```python
from build123d import *

# Parameters (mm, degrees)
SKETCH_1_W          = 84
SKETCH_1_H          = 55
EXTRUDE_2_DEPTH     = 8.5
EXTRUDE_3_DEPTH     = 5
SKETCH_2_W          = 84
SKETCH_2_H          = 3
CUT_EXTRUDE_1_DEPTH = 2


with BuildPart() as part:
    # Sketch 1 → Extrude 2 (new body)
    with BuildSketch(Plane.XY):
        Rectangle(SKETCH_1_W, SKETCH_1_H)
    extrude(amount=EXTRUDE_2_DEPTH)

    # Sketch 1_3 → Extrude 3 (add)
    with BuildSketch(Plane.XY):
        with BuildLine():
            Line((-29, 27.5), (-25, 27.5))
            ThreePointArc((-25, 27.5), (-27, 29.5), (-29, 27.5))
        make_face()
        with BuildLine():
            ThreePointArc((-42, 24.5), (-44, 22.5), (-42, 20.5))
            Line((-42, 20.5), (-42, 24.5))
        make_face()
        with BuildLine():
            ThreePointArc((-42, 2), (-44, 0), (-42, -2))
            Line((-42, -2), (-42, 2))
        make_face()
        with BuildLine():
            ThreePointArc((-42, -20.5), (-44, -22.5), (-42, -24.5))
            Line((-42, -24.5), (-42, -20.5))
        make_face()
        with BuildLine():
            Line((25, 27.5), (29, 27.5))
            ThreePointArc((29, 27.5), (27, 29.5), (25, 27.5))
        make_face()
    extrude(amount=EXTRUDE_3_DEPTH)

    # Sketch 2 → Cut-Extrude 1 (cut)
    with BuildSketch(Plane.XY.offset(8.5)):
        Rectangle(SKETCH_2_W, SKETCH_2_H)
    extrude(amount=-CUT_EXTRUDE_1_DEPTH, mode=Mode.SUBTRACT)


solid = part.part
```
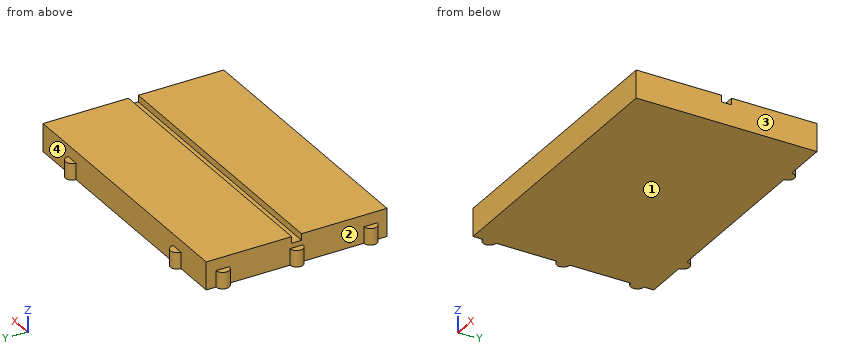
Geometry: final body of the model. Coordinates: model frame, mm. Face numbers are marked on the shaded views. Round coordinates to 2 decimals unless told otherwise and drop trailing zeros. Order: outer loops, then holes, each group sorted by start corner. A loop starts at its lowest first (then second) coordinate and runs counter-clockwise, first axis right, second up. Notation, with made-up numbers: (-9.5, 89.25) -> (11.5, 89.25) arc R25 cw to (11.5, 108.25) -> close; hole circle Ø4 at (89.25, -4.5). An arc over 180 degrees is marked (long way). Use one line per item in the form item = value.
(1) Draft query along X for the marked faces 1, 2, 3 and 4. Return one class per face: pulls with the +X half, pulls with the -X half, needs draft (parallel to the pull), parting line crosses it, or undercut.
Results list:
face_1 = needs draft
face_2 = pulls with the -X half
face_3 = pulls with the +X half
face_4 = undercut
(2) First-contact query: pin 1 Ø5 at (x, z) = (-20.5, 3) entering from +Y; pin 2 Ø2 at (x, y) = (-42.5, 21.5) entering from +Z; pin 3 Ø4 at (y, z) = (-6, 5) entering from -X; pin 4 Ø1 at (x, y) = (-43.5, -22) entering from +Z. Flat tips, straight axial feed; report the tip coordinate or a pass-through.
Results list:
pin_1 = 27.5
pin_2 = 8.5
pin_3 = -42
pin_4 = 5
(3) Section C-C on y = 0. Return loops of the section in (x, z).
Results list:
outline = (-44, 0) -> (42, 0) -> (42, 6.5) -> (-42, 6.5) -> (-42, 5) -> (-44, 5) -> close
(4) Section A-A on x = -6.5. Return loops of the section in (y, z).
Results list:
outline = (-27.5, 0) -> (27.5, 0) -> (27.5, 8.5) -> (1.5, 8.5) -> (1.5, 6.5) -> (-1.5, 6.5) -> (-1.5, 8.5) -> (-27.5, 8.5) -> close
(5) Section D-D on x = -27. Return loops of the section in (y, z).
Results list:
outline = (-27.5, 0) -> (29.5, 0) -> (29.5, 5) -> (27.5, 5) -> (27.5, 8.5) -> (1.5, 8.5) -> (1.5, 6.5) -> (-1.5, 6.5) -> (-1.5, 8.5) -> (-27.5, 8.5) -> close
(6) Section B-B on z = 4. Return loops of the section in (x, y).
Results list:
outline = (-42, -27.5) -> (42, -27.5) -> (42, 27.5) -> (29, 27.5) arc R2 ccw to (25, 27.5) -> (-25, 27.5) arc R2 ccw to (-29, 27.5) -> (-42, 27.5) -> (-42, 24.5) arc R2 ccw to (-42, 20.5) -> (-42, 2) arc R2 ccw to (-42, -2) -> (-42, -20.5) arc R2 ccw to (-42, -24.5) -> close
(7) Ray query, probe 1 along X at (y, z) = (-8, 7.75); probe 2 along Y at (x, z) = (16.5, 3); probe 3 along Y at (x, z) = (-18, 6.75). Return the intervals inside material, ascending. Write a range as [from, to].
Results list:
probe_1 = [-42, 42]
probe_2 = [-27.5, 27.5]
probe_3 = [-27.5, -1.5], [1.5, 27.5]
